Can you work these out from the model? Positions are in its coordinate system, mm. Face numbers are marked on the shaded views. A direction names the side the tool comes from. Round coordinates to 2 decimals unless told otherwise and drop trailing zeros. Loops run counter-clockwise (first coordinate to the right, second up) from the corner with the lowest first, then second, coordinate; pieces in that order, holes last. Notation, with made-up numbers: (72, 62) -> (103, 62) arc R34 cw to (103, 95) -> close; hole circle Ø5 at (74, 68). An arc over 180 degrees is marked (long way). Use a Markdown table: item, result.
Autodesk Inventor part; units mm, degrees
ref_plane "YZ Plane" through (0, 0, 0) normal (1, 0, 0) x (0, 1, 0)
ref_plane "XZ Plane" through (0, 0, 0) normal (0, 1, 0) x (-1, 0, 0)
ref_plane "XY Plane" through (0, 0, 0) normal (0, 0, 1) x (1, 0, 0)
sketch "Skizze1" plane through (0, 0, 0) normal (0, 0, 1) x (1, 0, 0)
  line L0 (-8.0351, 5.2058) -> (8.7518, 5.2058)
  line L1 (8.7518, 5.2058) -> (8.7518, -6.1866)
  line L2 (8.7518, -6.1866) -> (-8.0351, -6.1866)
  line L3 (-8.0351, -6.1866) -> (-8.0351, 5.2058)
  point P0 (0, 0)
extrude "Extrusion1" add sketch "Skizze1" along normal blind 10
sketch "Skizze2" plane through (0, 0, 10) normal (0, 0, 1) x (1, 0, 0)
  point P0 (0, 0)
hole "Drill01" at (0, 0, 10) direction (0, 0, -1) diameter 3 depth 8 tip angle 120
hole "Drill02" at (8.7518, 1.5333, 3.6521) direction (-1, 0, 0) diameter 4 depth 4 tip angle 118 counterbore diameter 5 counterbore depth 2
hole "Drill03" at (-0.835, -6.1866, 6.5728) direction (0, 1, 0) diameter 5 depth 6 tip angle 118 counterbore diameter 7 counterbore depth 2
hole "Drill04" at (4.8061, -2.4326, 10) direction (0, 0, -1) diameter 2 depth 6 tip angle 118 countersink diameter 3.5 countersink angle 90
properties part number "FxDrill_02"
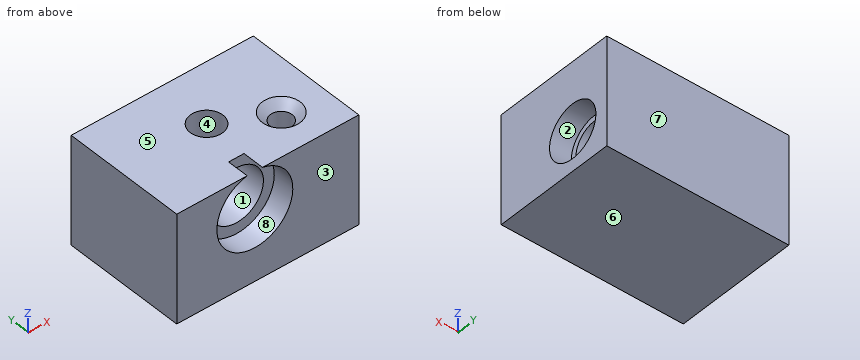
1. I want a section at C-C (y = -4.75). Please give me the cut outline in (x, z) (3 decimals), plus the area to 3 significant figures.
Answer sheet:
| item | result |
|---|---|
| outline | (-8.035, 0) -> (8.752, 0) -> (8.752, 10) -> (-0.125, 10) arc R3.5 cw (long way) to (-1.545, 10) -> (-8.035, 10) -> close |
| area | 129 mm² |
2. If we mould it in two halves opening along Z, with no side actions, what happens to the marked faces 5, 6, 7 and 8? For each: +Z half, -Z half, draft (parallel to the pull), parting line (faces both ways), or undercut.
Answer sheet:
| item | result |
|---|---|
| face 5 | +Z half |
| face 6 | -Z half |
| face 7 | draft |
| face 8 | undercut |
3. Which directions (+Z, -Z, +X, -X, +Y, -Y) give clear straight access to the entire face, cutting with the end or side of a thin tool? Please do the marked faces 1, 2, 3 and 4.
Answer sheet:
| item | result |
|---|---|
| face 1 | -Y |
| face 2 | +X |
| face 3 | +Z, -Z, +X, -X, -Y |
| face 4 | +Z |
4. I need wall thicknesses on line 1 (X direction, y = -3.25, z = 5.25); line 2 (Y direction, x = 0.25, z = 3.5); line 3 (X direction, y = 1.75, z = 1.5). Which ranges of each line are inside material? Lowest first, please.
Answer sheet:
| item | result |
|---|---|
| line 1 | x = -8.04 to -2.96, 1.29 to 4.23, 5.38 to 8.75 |
| line 2 | y = -4.19 to -1.48, 1.48 to 5.21 |
| line 3 | x = -8.04 to 6.75 |
5. I want a section at A-A (x = 2.25). Please give me the cut outline in (y, z), plus the area to 3 significant figures.
Answer sheet:
| item | result |
|---|---|
| outline | (-6.19, 0) -> (5.21, 0) -> (5.21, 10) -> (-6.19, 10) -> (-6.19, 8.23) -> (-4.19, 8.23) -> (-4.19, 4.92) -> (-6.19, 4.92) -> close |
| area | 107 mm² |
6. I want a section at B-B (x = 7). Please give me the cut outline in (y, z), plus the area to 3 significant figures.
Answer sheet:
| item | result |
|---|---|
| outline | (-6.19, 0) -> (5.21, 0) -> (5.21, 10) -> (-6.19, 10) -> close; hole circle Ø5 at (1.53, 3.65) |
| area | 94.3 mm² |
7. Will these pins go through, and if not, where does the flat tip stop? pin 1 Ø2.5 at (x, y) = (4.81, -2.43) entering from +Z; pin 2 Ø2.5 at (x, y) = (0, 0) entering from +Z.
Answer sheet:
| item | result |
|---|---|
| pin 1 | stops at z = 9.5 |
| pin 2 | stops at z = 1.86 |
